```python
from build123d import *

# Parameters (mm, degrees)
SKETCH1_W           = 300
SKETCH1_H           = 100
SKETCH1_R           = 20
BOSS_EXTRUDE1_DEPTH = 10
SKETCH2_W           = 300
SKETCH2_H           = 100
SKETCH2_W_2         = 280
SKETCH2_H_2         = 80
BOSS_EXTRUDE2_DEPTH = 50
SKETCH3_W           = 120
SKETCH3_H           = 30
BOSS_EXTRUDE3_DEPTH = 50
SKETCH4_W           = 120
SKETCH4_H           = 20
BOSS_EXTRUDE4_DEPTH = 19
SKETCH7_W           = 31
SKETCH7_H           = 30
BOSS_EXTRUDE5_DEPTH = 10
SKETCH8_W           = 31
SKETCH8_H           = 30
BOSS_EXTRUDE6_DEPTH = 10
SKETCH9_W           = 300
SKETCH9_H           = 100
SKETCH9_W_2         = 280
SKETCH9_H_2         = 80
BOSS_EXTRUDE7_DEPTH = 30


with BuildPart() as part:
    # Sketch1 → Boss-Extrude1 (new body)
    with BuildSketch(Plane.XY):
        Rectangle(SKETCH1_W, SKETCH1_H)
        with Locations((-85, 0)):
            Circle(SKETCH1_R, mode=Mode.SUBTRACT)
        with Locations((85, 0)):
            Circle(SKETCH1_R, mode=Mode.SUBTRACT)
    extrude(amount=BOSS_EXTRUDE1_DEPTH)

    # Sketch2 → Boss-Extrude2 (add)
    with BuildSketch(Plane(origin=(0, 0, 0), x_dir=(-1, 0, 0), z_dir=(0, 0, -1))):
        Rectangle(SKETCH2_W, SKETCH2_H)
        Rectangle(SKETCH2_W_2, SKETCH2_H_2, mode=Mode.SUBTRACT)
    extrude(amount=BOSS_EXTRUDE2_DEPTH)

    # Sketch3 → Boss-Extrude3 (add)
    with BuildSketch(Plane(origin=(0, 0, 0), x_dir=(-1, 0, 0), z_dir=(0, 0, -1))):
        with Locations((0, 25)):
            Rectangle(SKETCH3_W, SKETCH3_H)
        with Locations((0, -25)):
            Rectangle(SKETCH3_W, SKETCH3_H)
    extrude(amount=BOSS_EXTRUDE3_DEPTH)

    # Sketch4 → Boss-Extrude4 (add)
    with BuildSketch(Plane(origin=(0, 0, 0), x_dir=(-1, 0, 0), z_dir=(0, 0, -1))):
        Rectangle(SKETCH4_W, SKETCH4_H)
    extrude(amount=BOSS_EXTRUDE4_DEPTH)

    # Sketch7 → Boss-Extrude5 (add)
    with BuildSketch(Plane(origin=(60, 0, 0), x_dir=(0, 0, -1), z_dir=(1, 0, 0))):
        with Locations((34.5, 25)):
            Rectangle(SKETCH7_W, SKETCH7_H)
        with Locations((34.5, -25)):
            Rectangle(SKETCH7_W, SKETCH7_H)
    extrude(amount=BOSS_EXTRUDE5_DEPTH)

    # Sketch8 → Boss-Extrude6 (add)
    with BuildSketch(Plane.ZY.offset(60)):
        with Locations((-34.5, 25)):
            Rectangle(SKETCH8_W, SKETCH8_H)
        with Locations((-34.5, -25)):
            Rectangle(SKETCH8_W, SKETCH8_H)
    extrude(amount=BOSS_EXTRUDE6_DEPTH)

    # Sketch9 → Boss-Extrude7 (add)
    with BuildSketch(Plane(origin=(0, 0, -50), x_dir=(-1, 0, 0), z_dir=(0, 0, -1))):
        Rectangle(SKETCH9_W, SKETCH9_H)
        Rectangle(SKETCH9_W_2, SKETCH9_H_2, mode=Mode.SUBTRACT)
    extrude(amount=BOSS_EXTRUDE7_DEPTH)


solid = part.part
```
Geometry check sheet. Reference: the model listing, model coordinates, mm. A direction names the side the tool comes from. Coordinates: 2 decimals unless noted, no trailing zeros. Order: outer loops, then holes, each group sorted by start corner. A loop starts at its lowest first (then second) coordinate and runs counter-clockwise, first axis right, second up. Notation, with made-up numbers: (-31.5, -5.5) - (3.5, -5.5) arc R27 cw to (3.5, 25.5) - close; hole circle Ø6 at (-7, -32). An arc over 180 degrees is marked (long way). Use one line per item in the form item = value.
1. Section check B-B (x = -85). Record the boundary of the cut face in (y, z).
Here are the results:
outline = (-50, -80) - (-40, -80) - (-40, 0) - (-20, 0) - (-20, 10) - (-50, 10) - close; (20, 0) - (40, 0) - (40, -80) - (50, -80) - (50, 10) - (20, 10) - close
2. Section check A-A (y = 0). Record the boundary of the cut face in (x, z), then the cut area to 3 significant figures.
Here are the results:
outline = (-150, -80) - (-140, -80) - (-140, 0) - (-105, 0) - (-105, 10) - (-150, 10) - close; (-65, 0) - (-60, 0) - (-60, -19) - (60, -19) - (60, 0) - (65, 0) - (65, 10) - (-65, 10) - close; (105, 0) - (140, 0) - (140, -80) - (150, -80) - (150, 10) - (105, 10) - close
area = 6,080 mm²
3. Draft check along Y on faces 1 (the face through (12, -41, -80)), 2 (the face through (2, -50, -34)), 3 (the face through (-109, 1, 0)). Enter one of: pulls with the +Y half, pulls with the -Y half, needs draft (parallel to the pull), parting line crosses it, or undercut.
Here are the results:
face_1 = needs draft
face_2 = pulls with the -Y half
face_3 = undercut
4. Section check D-D (z = -71). Record the boundary of the cut face in (x, y), then the cut area to 3 significant figures.
Here are the results:
outline = (-150, -50) - (150, -50) - (150, 50) - (-150, 50) - close; hole (-140, -40) - (140, -40) - (140, 40) - (-140, 40) - close
area = 7,600 mm²
5. Scan lines: line 1 (Y direction, x = -85, z = 3); line 2 (X direction, y = -4.5, z = -61.5); line 3 (X direction, y = -18.5, z = -18). Record each from-to range of solid material in increasing order.
Here are the results:
line_1 = -50 to -20, 20 to 50
line_2 = -150 to -140, 140 to 150
line_3 = -150 to -140, -60 to 60, 140 to 150
6. Gauge pin test, flat ends, axial feed: pin 1 (24 mm diameter, centred on x = 117.5, y = -10, fed in from -Z); pin 2 (6 mm diameter, centred on x = 29.5, y = -3.5, fed in from -Z). Record the tip position at first contact, or that the pin passes through.
Here are the results:
pin_1 = 0
pin_2 = -19
7. Section check C-C (y = 27). Record the boundary of the cut face in (x, z), then the cut area to 3 significant figures.
Here are the results:
outline = (-150, -80) - (-140, -80) - (-140, 0) - (-60, 0) - (-60, -19) - (-70, -19) - (-70, -50) - (70, -50) - (70, -19) - (60, -19) - (60, 0) - (140, 0) - (140, -80) - (150, -80) - (150, 10) - (-150, 10) - close
area = 11,200 mm²
8. Access from +Z, -Z, +X, -X, +Y, -Y to the whole of each face (thin tool, end or side, straight path). Record for faces 4 (the face through (65, -25, -19)), 5 (the face through (-140, -1, -39)), 6 (the face through (-150, -1, -34)).
Here are the results:
face_4 = none
face_5 = -Z
face_6 = +Z, -Z, -X, +Y, -Y
